Build history of the part. All positions in model axes, mm. A direction names the side the tool comes from. Coordinates: 2 decimals unless noted, no trailing zeros. Write each loop counter-clockwise with the first axis right and the second up, starting at its lowest first coordinate (ties: lowest second). Pieces come first, ordered by that corner, then holes. Notation, with made-up numbers: (34, -21) -> (42, -21) arc R24 ccw to (42, -1) -> close; hole circle Ø7 at (87.5, 86.5). An arc over 180 degrees is marked (long way). Write each question's results on one line, items separated by ' | '. Start each with the question number.
Q1. Saw through at B-B on x = -4. Give the cut face in (y, z).
Q2. Drill centre lines: line 1 (Y direction, x = -11, z = 8); line 2 (Y direction, x = -44, z = -83); line 3 (Z direction, x = -9.5, y = -4). Where is each one in solid material? Low to high.
Q3. Saw through at D-D on y = 14.5. Give the cut face in (x, z).
Q4. Saw through at A-A on y = -2. Give the cut face in (x, z), and give its area (3 significant figures).
Q5. Tool access for faces 1 (the face through (-1, -14, -20)), 2 (the face through (-25, 0, -85)), 3 (the face through (-1, 14, -20)), 4 (the face through (12, -10, -80)): list every direction of +Z, -Z, +X, -X, +Y, -Y with a clear straight run to the whole face (end or side of a thin tool).
Q6. Saw through at C-C on z = 2. Give the cut face in (x, y), and give its area (3 significant figures).
Q7. Two-plate mould, pull along Z, no slides. Class faces 5 (the face through (-25, -10, -100)), 6 (the face through (0, 0, 20)), 7 (the face through (-47, -7, -40)), 8 (the face through (25, 0, -85)): released by +Z, released by -Z, zero draft, split by the parting line, or undercut.
Q8. Drop flat-ended pins along their axis: pin 1 Ø6 at (x, y) = (-0.5, 13.5) entering from +Z; pin 2 Ø5.5 at (y, z) = (-18, -39) entering from -X; pin 3 Ø8 at (x, z) = (25, -86.5) entering from +Y. Give the stop position or say it passes through.
from build123d import *

# Parameters (mm, degrees)
EXTRUDE_1_DEPTH     = 20
SKETCH_2_W          = 106.736402143
SKETCH_2_H          = 47.429352318
CUT_EXTRUDE_1_DEPTH = 12
SKETCH_3_W          = 102.678215223
SKETCH_3_H          = 46.458192726
CUT_EXTRUDE_2_DEPTH = 12
CUT_EXTRUDE_3_DEPTH = 130.614813968
CUT_EXTRUDE_4_DEPTH = 16
EXTRUDE_4_DEPTH     = 100
SKETCH_8_W          = 10
SKETCH_8_H          = 20
CUT_EXTRUDE_6_DEPTH = 100
CUT_EXTRUDE_7_DEPTH = 16


with BuildPart() as part:
    # 草图1 → 凸台-拉伸1 (new, symmetric)
    with BuildSketch(Plane(origin=(0, 0, 0), x_dir=(1, 0, 0), z_dir=(0, 1, 0))):
        with BuildLine():
            Line((-50, 20), (-13.793103448, -14.482758621))
            ThreePointArc((-13.793103448, -14.482758621), (0, -20), (13.793103448, -14.482758621))
            Line((13.793103448, -14.482758621), (50, 20))
            Line((50, 20), (50, 80))
            Line((50, 80), (-50, 80))
            Line((-50, 80), (-50, 20))
        make_face()
    extrude(amount=EXTRUDE_1_DEPTH, both=True)

    # 草图2 → 切除-拉伸1 (cut)
    with BuildSketch(Plane(origin=(0, 20, 0), x_dir=(1, 0, 0), z_dir=(0, 1, 0))):
        with Locations((3.368201072, -3.714676159)):
            Rectangle(SKETCH_2_W, SKETCH_2_H)
    extrude(amount=-CUT_EXTRUDE_1_DEPTH, mode=Mode.SUBTRACT)

    # 草图3 → 切除-拉伸2 (cut)
    with BuildSketch(Plane.XZ.offset(20)):
        with Locations((1.339107612, 3.229096363)):
            Rectangle(SKETCH_3_W, SKETCH_3_H)
    extrude(amount=-CUT_EXTRUDE_2_DEPTH, mode=Mode.SUBTRACT)

    # 草图4 → 切除-拉伸3 (cut, through all)
    with BuildSketch(Plane(origin=(50, 0, 0), x_dir=(0, 0, -1), z_dir=(1, 0, 0))):
        Polygon((80, 0), (50, 20), (88.61691531, 20), (88.61691531, 0), align=None)
    extrude(amount=-CUT_EXTRUDE_3_DEPTH, mode=Mode.SUBTRACT)

    # Sketch 3D_1 → 切除-拉伸4 (cut)
    with BuildSketch(Plane(origin=(37, -14.910720316, -32), x_dir=(0.9127147422515467, 0.40859735593453445, 0), z_dir=(0, 0, -1))):
        with BuildLine():
            Line((0, 0), (-3.444952044, 7.6952493))
            Line((-3.444952044, 7.6952493), (4.401902282, 10.724720717))
            ThreePointArc((4.401902282, 10.724720717), (10.279015254, 10.694120637), (14.549253267, 6.655994763))
            Line((14.549253267, 6.655994763), (19.7295953, 0))
            Line((19.7295953, 0), (10.525702717, -4.05282768))
            ThreePointArc((10.525702717, -4.05282768), (4.4271171, -4.196920719), (0, 0))
        make_face()
    extrude(amount=CUT_EXTRUDE_4_DEPTH, mode=Mode.SUBTRACT)

    # 草图6 → 凸台-拉伸4 (add)
    with BuildSketch(Plane.ZY.offset(50)):
        with BuildLine():
            Line((-90, 0), (-80, 0))
            Line((-80, 0), (-80, -20))
            Line((-80, -20), (-90, -20))
            ThreePointArc((-90, -20), (-100, -10), (-90, 0))
        make_face()
    extrude(amount=-EXTRUDE_4_DEPTH)

    # 草图8 → 切除-拉伸6 (cut)
    with BuildSketch(Plane.XZ.offset(20)):
        with Locations((-37.5, -90)):
            Rectangle(SKETCH_8_W, SKETCH_8_H)
        with Locations((-12.5, -90)):
            Rectangle(SKETCH_8_W, SKETCH_8_H)
        with Locations((12.5, -90)):
            Rectangle(SKETCH_8_W, SKETCH_8_H)
        with Locations((37.5, -90)):
            Rectangle(SKETCH_8_W, SKETCH_8_H)
    extrude(amount=-CUT_EXTRUDE_6_DEPTH, mode=Mode.SUBTRACT)

    # 草图9 → 切除-拉伸7 (cut)
    with BuildSketch(Plane(origin=(0, 0, -32), x_dir=(-1, 0, 0), z_dir=(0, 0, -1))):
        with BuildLine():
            Line((45, -7), (50, -7))
            Line((50, -7), (59.459591305, -7))
            Line((59.459591305, -7), (59.459591305, -23))
            Line((59.459591305, -23), (37, -23))
            Line((37, -23), (37, -15))
            ThreePointArc((37, -15), (39.343145751, -9.343145751), (45, -7))
        make_face()
    extrude(amount=CUT_EXTRUDE_7_DEPTH, mode=Mode.SUBTRACT)


solid = part.part
Returned:
1) outline: (-20, -90) arc R10 ccw to (0, -90) -> (0, -80) -> (20, -50) -> (20, -20) -> (8, -20) -> (8, 19.6) -> (-8, 19.6) -> (-8, -20) -> (-20, -20) -> close
2) line 1: y = -8 to 8 | line 2: y = -20 to 0 | line 3: z = -80 to 17.6
3) outline: (-50, -58.25) -> (50, -58.25) -> (50, -20) -> (-50, -20) -> close
4) outline: (-50, -96) -> (-42.5, -96) -> (-42.5, -80) -> (-32.5, -80) -> (-32.5, -96) -> (-17.5, -96) -> (-17.5, -80) -> (-7.5, -80) -> (-7.5, -96) -> (7.5, -96) -> (7.5, -80) -> (17.5, -80) -> (17.5, -96) -> (32.5, -96) -> (32.5, -80) -> (42.5, -80) -> (42.5, -96) -> (50, -96) -> (50, -20) -> (13.79, 14.48) arc R20 ccw to (-13.79, 14.48) -> (-50, -20) -> close | area: 9,260 mm2
5) face 1: +Z, +X, -X, -Y | face 2: -Z, +X, -X, +Y | face 3: +Z, +X, -X, +Y | face 4: -Z, +Y, -Y
6) outline: (-26.9, -8) -> (26.9, -8) -> (26.9, 8) -> (-26.9, 8) -> close | area: 861 mm2
7) face 5: released by -Z | face 6: released by +Z | face 7: undercut | face 8: zero draft
8) pin 1: stops at z = -20 | pin 2: stops at x = -37 | pin 3: stops at y = 0
